The listing builds one solid part. Answer for the finished solid, in the listing's coordinates (mm). Round coordinates to 2 decimals unless told otherwise and drop trailing zeros. Write each loop counter-clockwise with the first axis right and the second up, starting at its lowest first coordinate (ties: lowest second). Pieces come first, ordered by that corner, then holes. Notation, with made-up numbers: M 89,24 L 146,24 A20 ccw 146,34 Z; hole C 13,63 d2. An arc over 180 degrees is marked long. Answer as CSV lines item,"result". Start each with the question number.
from build123d import *

# Parameters (mm, degrees)
SKETCH2_W           = 49.736379614
SKETCH2_H           = 50
BOSS_EXTRUDE2_DEPTH = 1
SKETCH3_R           = 19.5
CUT_EXTRUDE1_DEPTH  = 1
SKETCH6_R           = 1.8
CUT_EXTRUDE2_DEPTH  = 2


with BuildPart() as part:
    # Sketch2 → Boss-Extrude2 (new body)
    with BuildSketch(Plane.XY):
        Rectangle(SKETCH2_W, SKETCH2_H)
    extrude(amount=BOSS_EXTRUDE2_DEPTH)

    # Sketch3 → Cut-Extrude1 (cut)
    with BuildSketch(Plane.XY.offset(1)):
        with Locations((0, -1.3)):
            Circle(SKETCH3_R)
    extrude(amount=-CUT_EXTRUDE1_DEPTH, mode=Mode.SUBTRACT)

    # Sketch6 → Cut-Extrude2 (cut, through all)
    with BuildSketch(Plane.XY.offset(1)):
        with Locations((-15.908992298, 14.714110903)):
            Circle(SKETCH6_R)
        with Locations((16.091007702, 14.714110903)):
            Circle(SKETCH6_R)
    extrude(amount=-CUT_EXTRUDE2_DEPTH, mode=Mode.SUBTRACT)


solid = part.part
Q1. Find section B-B (y = -1.3). Determine the outline of the cut face in (x, z), plus the area to 3 significant figures.
Q2. Find section A-A (x = 0). Determine the outline of the cut face in (y, z).
Q3. Straight lines are drawn through the part: L1, parallel to Y at x = -16.5, z = 0.65; L2, parallel to Y at x = 0, z = 0.4; L3, parallel to X at y = -3.5, z = 0.55. For each, find the intervals that lie inside material, in ascending order.
Q4. The mould has two halves that part along X. Classify faces 1 (the face through (9, -18.6, 0.5)), 2 (the face through (-11, 17, 0)): +X half, -X half, draft (parallel to the pull), parting line (faces both ways), or undercut.
Q5. Find section C-C (z = 0.75). Determine the outline of the cut face in (x, y), plus the area to 3 significant figures.
Q6. This flat-tipped pin is pushed along its axis until it touches: P1, Ø4.5, axis at x = -15.91, y = 14.71, coming from the +Z side. Where does it stop, or does it pass through?
Reported:
1,outline,"M -24.87,0 L -19.5,0 L -19.5,1 L -24.87,1 Z; M 19.5,0 L 24.87,0 L 24.87,1 L 19.5,1 Z"
1,area,"10.7 mm2"
2,outline,"M -25,0 L -20.8,0 L -20.8,1 L -25,1 Z; M 18.2,0 L 25,0 L 25,1 L 18.2,1 Z"
3,L1,"y = -25 to -11.69, 9.09 to 13.01, 16.41 to 25"
3,L2,"y = -25 to -20.8, 18.2 to 25"
3,L3,"x = -24.87 to -19.38, 19.38 to 24.87"
4,face 1,"undercut"
4,face 2,"draft"
5,outline,"M -24.87,-25 L 24.87,-25 L 24.87,25 L -24.87,25 Z; hole C 0,-1.3 d39; hole C -15.91,14.71 d3.6; hole C 16.09,14.71 d3.6"
5,area,"1,270 mm2"
6,P1,"stops at z = 1"
